from build123d import *

# Parameters (mm, degrees)
SKETCH1_R           = 3.3782
SKETCH1_R_2         = 6.35
BOSS_EXTRUDE1_DEPTH = 1.5875
FILLET1_R           = 12.7


with BuildPart() as part:
    # Sketch1 → Boss-Extrude1 (new, symmetric)
    with BuildSketch(Plane(origin=(0, 0, 0), x_dir=(0, 0, -1), z_dir=(1, 0, 0))):
        with BuildLine():
            Line((0, 0), (0, 203.2))
            Line((0, 203.2), (-209.55, 203.2))
            Line((-209.55, 203.2), (-209.55, 25.4))
            Line((-209.55, 25.4), (-184.15, 0))
            Line((-184.15, 0), (-98.425, 0))
            ThreePointArc((-98.425, 0), (-96.17993597, 0.92993597), (-95.25, 3.175))
            Line((-95.25, 3.175), (-95.25, 12.7))
            ThreePointArc((-95.25, 12.7), (-88.9, 19.05), (-82.55, 12.7))
            Line((-82.55, 12.7), (-82.55, 3.175))
            ThreePointArc((-82.55, 3.175), (-81.62006403, 0.92993597), (-79.375, 0))
            Line((-79.375, 0), (0, 0))
        make_face()
        with Locations((-12.7, 12.7)):
            Circle(SKETCH1_R, mode=Mode.SUBTRACT)
        with Locations((-63.5, 12.7)):
            Circle(SKETCH1_R, mode=Mode.SUBTRACT)
        with Locations((-114.3, 12.7)):
            Circle(SKETCH1_R, mode=Mode.SUBTRACT)
        with Locations((-12.7, 85.725)):
            Circle(SKETCH1_R, mode=Mode.SUBTRACT)
        with Locations((-38.1, 85.725)):
            Circle(SKETCH1_R, mode=Mode.SUBTRACT)
        with Locations((-63.5, 85.725)):
            Circle(SKETCH1_R, mode=Mode.SUBTRACT)
        with Locations((-88.9, 85.725)):
            Circle(SKETCH1_R, mode=Mode.SUBTRACT)
        with Locations((-12.7, 184.15)):
            Circle(SKETCH1_R_2, mode=Mode.SUBTRACT)
        with Locations((-38.1, 184.15)):
            Circle(SKETCH1_R_2, mode=Mode.SUBTRACT)
        with Locations((-63.5, 184.15)):
            Circle(SKETCH1_R_2, mode=Mode.SUBTRACT)
        with Locations((-88.9, 184.15)):
            Circle(SKETCH1_R_2, mode=Mode.SUBTRACT)
        with Locations((-114.3, 184.15)):
            Circle(SKETCH1_R_2, mode=Mode.SUBTRACT)
        with Locations((-190.5, 184.15)):
            Circle(SKETCH1_R_2, mode=Mode.SUBTRACT)
        with Locations((-139.7, 12.7)):
            Circle(SKETCH1_R, mode=Mode.SUBTRACT)
        with Locations((-165.1, 12.7)):
            Circle(SKETCH1_R, mode=Mode.SUBTRACT)
        with Locations((-114.3, 85.725)):
            Circle(SKETCH1_R, mode=Mode.SUBTRACT)
        with Locations((-139.7, 85.725)):
            Circle(SKETCH1_R, mode=Mode.SUBTRACT)
        with Locations((-165.1, 85.725)):
            Circle(SKETCH1_R, mode=Mode.SUBTRACT)
        with Locations((-190.5, 85.725)):
            Circle(SKETCH1_R, mode=Mode.SUBTRACT)
        with BuildLine():
            Line((-76.2, 73.025), (-76.2, 25.4))
            ThreePointArc((-76.2, 25.4), (-75.27006403, 23.15493597), (-73.025, 22.225))
            Line((-73.025, 22.225), (-47.625, 22.225))
            Line((-47.625, 22.225), (-47.625, 19.05))
            ThreePointArc((-47.625, 19.05), (-38.1, 9.525), (-28.575, 19.05))
            Line((-28.575, 19.05), (-28.575, 22.225))
            ThreePointArc((-28.575, 22.225), (-26.32993597, 23.15493597), (-25.4, 25.4))
            Line((-25.4, 25.4), (-25.4, 73.025))
            ThreePointArc((-25.4, 73.025), (-26.32993597, 75.27006403), (-28.575, 76.2))
            Line((-28.575, 76.2), (-73.025, 76.2))
            ThreePointArc((-73.025, 76.2), (-75.27006403, 75.27006403), (-76.2, 73.025))
        make_face(mode=Mode.SUBTRACT)
        with BuildLine():
            Line((-33.945106311, 104.775), (-53.975, 104.775))
            ThreePointArc((-53.975, 104.775), (-56.22006403, 105.70493597), (-57.15, 107.95))
            Line((-57.15, 107.95), (-57.15, 150.012776746))
            ThreePointArc((-57.15, 150.012776746), (-54.674723761, 153.109712596), (-51.108417853, 151.377815864))
            Line((-51.108417853, 151.377815864), (-31.078524164, 109.315039118))
            ThreePointArc((-31.078524164, 109.315039118), (-31.260462555, 106.254915076), (-33.945106311, 104.775))
        make_face(mode=Mode.SUBTRACT)
        with BuildLine():
            Line((-25.4, 133.597084881), (-25.4, 168.275))
            ThreePointArc((-25.4, 168.275), (-26.32993597, 170.52006403), (-28.575, 171.45))
            Line((-28.575, 171.45), (-45.088292914, 171.45))
            ThreePointArc((-45.088292914, 171.45), (-47.77293667, 169.970084924), (-47.954875061, 166.909960882))
            Line((-47.954875061, 166.909960882), (-31.441582147, 132.232045763))
            ThreePointArc((-31.441582147, 132.232045763), (-27.875276239, 130.500149031), (-25.4, 133.597084881))
        make_face(mode=Mode.SUBTRACT)
        with BuildLine():
            Line((-180.364167607, 23.15493597), (-189.57006403, 32.360832393))
            ThreePointArc((-189.57006403, 32.360832393), (-190.258317516, 33.390876526), (-190.5, 34.605896424))
            Line((-190.5, 34.605896424), (-190.5, 73.025))
            ThreePointArc((-190.5, 73.025), (-189.57006403, 75.27006403), (-187.325, 76.2))
            Line((-187.325, 76.2), (-104.775, 76.2))
            ThreePointArc((-104.775, 76.2), (-102.52993597, 75.27006403), (-101.6, 73.025))
            Line((-101.6, 73.025), (-101.6, 25.4))
            ThreePointArc((-101.6, 25.4), (-102.52993597, 23.15493597), (-104.775, 22.225))
            Line((-104.775, 22.225), (-178.119103576, 22.225))
            ThreePointArc((-178.119103576, 22.225), (-179.334123474, 22.466682484), (-180.364167607, 23.15493597))
        make_face(mode=Mode.SUBTRACT)
        with BuildLine():
            Line((-79.045124939, 166.909960882), (-95.558417853, 132.232045763))
            ThreePointArc((-95.558417853, 132.232045763), (-99.124723761, 130.500149031), (-101.6, 133.597084881))
            Line((-101.6, 133.597084881), (-101.6, 168.275))
            ThreePointArc((-101.6, 168.275), (-100.67006403, 170.52006403), (-98.425, 171.45))
            Line((-98.425, 171.45), (-81.911707086, 171.45))
            ThreePointArc((-81.911707086, 171.45), (-79.22706333, 169.970084924), (-79.045124939, 166.909960882))
        make_face(mode=Mode.SUBTRACT)
        with BuildLine():
            Line((-75.891582147, 151.377815864), (-95.921475836, 109.315039118))
            ThreePointArc((-95.921475836, 109.315039118), (-95.739537445, 106.254915076), (-93.054893689, 104.775))
            Line((-93.054893689, 104.775), (-73.025, 104.775))
            ThreePointArc((-73.025, 104.775), (-70.77993597, 105.70493597), (-69.85, 107.95))
            Line((-69.85, 107.95), (-69.85, 150.012776746))
            ThreePointArc((-69.85, 150.012776746), (-72.325276239, 153.109712596), (-75.891582147, 151.377815864))
        make_face(mode=Mode.SUBTRACT)
        with BuildLine():
            Line((-122.845106311, 104.775), (-142.875, 104.775))
            ThreePointArc((-142.875, 104.775), (-145.12006403, 105.70493597), (-146.05, 107.95))
            Line((-146.05, 107.95), (-146.05, 150.012776746))
            ThreePointArc((-146.05, 150.012776746), (-143.574723761, 153.109712596), (-140.008417853, 151.377815864))
            Line((-140.008417853, 151.377815864), (-119.978524164, 109.315039118))
            ThreePointArc((-119.978524164, 109.315039118), (-120.160462555, 106.254915076), (-122.845106311, 104.775))
        make_face(mode=Mode.SUBTRACT)
        with BuildLine():
            Line((-114.3, 133.597084881), (-114.3, 168.275))
            ThreePointArc((-114.3, 168.275), (-115.22993597, 170.52006403), (-117.475, 171.45))
            Line((-117.475, 171.45), (-133.988292914, 171.45))
            ThreePointArc((-133.988292914, 171.45), (-136.67293667, 169.970084924), (-136.854875061, 166.909960882))
            Line((-136.854875061, 166.909960882), (-120.341582147, 132.232045763))
            ThreePointArc((-120.341582147, 132.232045763), (-116.775276239, 130.500149031), (-114.3, 133.597084881))
        make_face(mode=Mode.SUBTRACT)
        with BuildLine():
            Line((-167.945124939, 166.909960882), (-184.458417853, 132.232045763))
            ThreePointArc((-184.458417853, 132.232045763), (-188.024723761, 130.500149031), (-190.5, 133.597084881))
            Line((-190.5, 133.597084881), (-190.5, 168.275))
            ThreePointArc((-190.5, 168.275), (-189.57006403, 170.52006403), (-187.325, 171.45))
            Line((-187.325, 171.45), (-170.811707086, 171.45))
            ThreePointArc((-170.811707086, 171.45), (-168.12706333, 169.970084924), (-167.945124939, 166.909960882))
        make_face(mode=Mode.SUBTRACT)
        with BuildLine():
            Line((-164.791582147, 151.377815864), (-184.821475836, 109.315039118))
            ThreePointArc((-184.821475836, 109.315039118), (-184.639537445, 106.254915076), (-181.954893689, 104.775))
            Line((-181.954893689, 104.775), (-161.925, 104.775))
            ThreePointArc((-161.925, 104.775), (-159.67993597, 105.70493597), (-158.75, 107.95))
            Line((-158.75, 107.95), (-158.75, 150.012776746))
            ThreePointArc((-158.75, 150.012776746), (-161.225276239, 153.109712596), (-164.791582147, 151.377815864))
        make_face(mode=Mode.SUBTRACT)
        with BuildLine():
            Line((-133.35, 177.8), (-171.45, 177.8))
            ThreePointArc((-171.45, 177.8), (-177.8, 184.15), (-171.45, 190.5))
            Line((-171.45, 190.5), (-133.35, 190.5))
            ThreePointArc((-133.35, 190.5), (-127, 184.15), (-133.35, 177.8))
        make_face(mode=Mode.SUBTRACT)
    extrude(amount=BOSS_EXTRUDE1_DEPTH, both=True)

    # Fillet1
    fillet1_edges = [part.edges().sort_by_distance(p)[0] for p in [
        (0, 0, 184.15),
        (0, 25.4, 209.55),
        (0, 203.2, 209.55),
        (0, 203.2, 0),
        (0, 0, 0),
    ]]
    fillet(fillet1_edges, radius=FILLET1_R)


solid = part.part
Build history of the part. All positions in model axes, mm. Coordinates: 2 decimals unless noted, no trailing zeros. Write each loop counter-clockwise with the first axis right and the second up, starting at its lowest first coordinate (ties: lowest second). Pieces come first, ordered by that corner, then holes. Notation, with made-up numbers: (1.25, 28.5) -> (47.25, 28.5) arc R14 cw to (47.25, 46.5) -> close; hole circle Ø9 at (38, -34). An arc over 180 degrees is marked (long way). Use CSV: the item, a comma, the result in double quotes. Start each with the question number.
Q1. Cut at D-D, the plane y = 163. List the corners of the cut face in (x, z).
Q2. Drill centre lines: probe 1 along Z at (x, y) = (0.9, 52.5); probe 2 along Y at (x, z) = (0.5, 12.7); probe 3 along Y at (x, z) = (0.9, 88.9) (3 decimals). Where is each one in solid material? Low to high.
Q3. Cut at B-B, the plane z = 63.5. List the corners of the cut face in (x, y) (1 decimal).
Q4. Cut at C-C, the plane y = 59.5. List the corners of the cut face in (x, z).
Q5. Flat gauge pin, fed straight in: pin 1 Ø1 at (x, y) = (-0.5, 10) entering from +Z. Where does the tip first touch, or does it go through?
Q6. Cut at A-A, the plane y = 184.15. State how many separate pieces and enclosed holes the cut face has, then the cut area to 3 significant figures.
Q7. Pull direction Z, two halves, no side cores. Call faces 1 (the cylindrical face through (0.02, 199.38, 3.62)), 2 (the flat face through (0.022, 130.641, 130.134)), 3 (the cylindrical face through (0, 178.5, 111.4)), 4 (the flat face through (1.588, 126, 106)): released by +Z, released by -Z, zero draft, split by the parting line, or undercut.
Checked values:
1,outline,"(-1.59, 0) -> (1.59, 0) -> (1.59, 25.4) -> (-1.59, 25.4) -> close; (-1.59, 46.09) -> (1.59, 46.09) -> (1.59, 80.91) -> (-1.59, 80.91) -> close; (-1.59, 101.6) -> (1.59, 101.6) -> (1.59, 114.3) -> (-1.59, 114.3) -> close; (-1.59, 134.99) -> (1.59, 134.99) -> (1.59, 169.81) -> (-1.59, 169.81) -> close; (-1.59, 190.5) -> (1.59, 190.5) -> (1.59, 209.55) -> (-1.59, 209.55) -> close"
2,probe 1,"z = 0 to 25.4, 76.2 to 101.6, 190.5 to 209.55"
2,probe 2,"y = 0 to 9.32, 16.08 to 82.35, 89.1 to 177.8, 190.5 to 203.2"
2,probe 3,"y = 19.05 to 82.347, 89.103 to 104.775, 124.06 to 146.215, 171.45 to 177.8, 190.5 to 203.2"
3,outline,"(-1.6, 0) -> (1.6, 0) -> (1.6, 9.3) -> (-1.6, 9.3) -> close; (-1.6, 16.1) -> (1.6, 16.1) -> (1.6, 22.2) -> (-1.6, 22.2) -> close; (-1.6, 76.2) -> (1.6, 76.2) -> (1.6, 82.3) -> (-1.6, 82.3) -> close; (-1.6, 89.1) -> (1.6, 89.1) -> (1.6, 177.8) -> (-1.6, 177.8) -> close; (-1.6, 190.5) -> (1.6, 190.5) -> (1.6, 203.2) -> (-1.6, 203.2) -> close"
4,outline,"(-1.59, 0) -> (1.59, 0) -> (1.59, 25.4) -> (-1.59, 25.4) -> close; (-1.59, 76.2) -> (1.59, 76.2) -> (1.59, 101.6) -> (-1.59, 101.6) -> close; (-1.59, 190.5) -> (1.59, 190.5) -> (1.59, 209.55) -> (-1.59, 209.55) -> close"
5,pin 1,"stops at z = 194.65"
6,separate pieces,"8"
6,enclosed holes,"0"
6,area,"262 mm²"
7,face 1,"released by -Z"
7,face 2,"undercut"
7,face 3,"undercut"
7,face 4,"zero draft"
